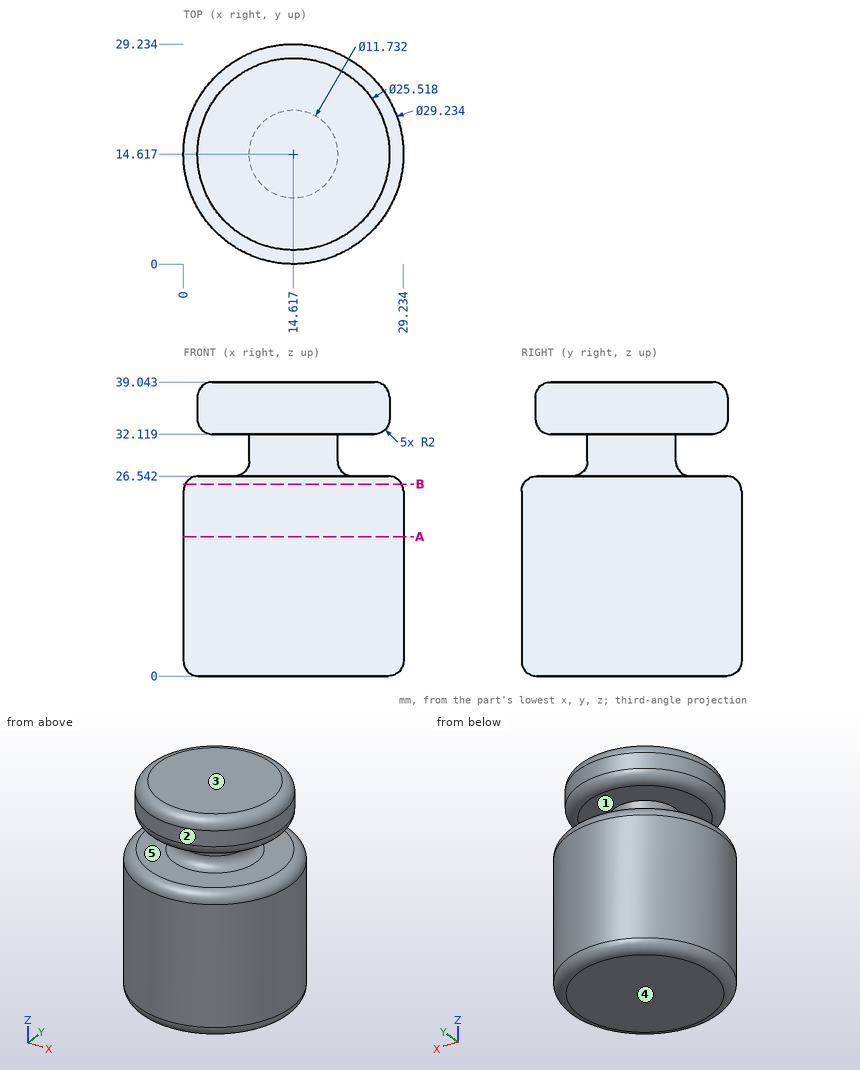
Can you work these out from the drawing? Everything is in mm from the part's minimum corner. A direction names the side the tool comes from. Round coordinates to 2 decimals unless told otherwise and drop trailing zeros. Loops run counter-clockwise (first coordinate to the right, second up) from the corner with the lowest first, then second, coordinate; pieces in that order, holes last. Notation, with made-up numbers: M -24,-5 L -14,-5 A29 cw -14,31 Z; hole C 23.25,15.5 d7. An arc over 180 degrees is marked long. Answer in a Markdown table with one row per item.
1. Thinking about a two-plate mould opening in Z: for the marked faces 1, 2 and 3, which applies, pulls with the +Z half, pulls with the -Z half, needs draft (parallel to the pull), parting line crosses it, or undercut?
Established:
| item | result |
|---|---|
| face 1 | undercut |
| face 2 | needs draft |
| face 3 | pulls with the +Z half |
2. If we section it at B-B, the plane z = 25.5: Please give me the cut outline in (x, y) (1 decimal).
Established:
| item | result |
|---|---|
| outline | C 14.6,14.6 d28.7 |
3. On a 3-axis mill with a long thin cutter (end or side, diameter ignored), from which of +Z, -Z, +X, -X, +Y, -Y can I reach the whole of each face in a straight line? I mean the marked faces 4 and 5. Say none if no direction works.
Established:
| item | result |
|---|---|
| face 4 | -Z, +X, -X, +Y, -Y |
| face 5 | none |
4. If we section it at A-A, the plane z = 18.5: Please give me the cut outline in (x, y) (1 decimal).
Established:
| item | result |
|---|---|
| outline | C 14.6,14.6 d29.2 |
5. Please list where these lines run through material, in increasing order: line 1 (Z direction, x = 6.5, y = 9.5); line 2 (Z direction, x = 26.75, y = 12) (1 decimal); line 3 (Y direction, x = 8.25, z = 5) (1 decimal). Write a range as from..to.
Established:
| item | result |
|---|---|
| line 1 | 0..26.54, 32.12..39.04 |
| line 2 | 0..26.5, 33..38.2 |
| line 3 | 1.5..27.8 |
6. I'm going to push flat-ended pins straight in: pin 1 Ø5 at (x, z) = (11, 34) entering from +Y; pin 2 Ø1 at (x, z) = (22.5, 30.5) entering from +Y; pin 3 Ø1.5 at (x, z) = (9.5, 22) entering from +Y; pin 4 Ø10 at (x, z) = (9, 8.5) entering from -Y. Where does each tip first touch, or does it pass through?
Established:
| item | result |
|---|---|
| pin 1 | y = 27.33 |
| pin 2 | through |
| pin 3 | y = 28.57 |
| pin 4 | y = 0.01 |
